Could you check a few things on this model? Use its own coordinates, in mm. A direction names the side the tool comes from. Coordinates: 2 decimals unless noted, no trailing zeros. Order: outer loops, then holes, each group sorted by start corner. A loop starts at its lowest first (then second) coordinate and runs counter-clockwise, first axis right, second up. Notation, with made-up numbers: M -8.5,46 L 34.5,46 A16 ccw 34.5,72 Z; hole C 85,56 d2. An arc over 180 degrees is marked long. Put each result on its own line as item: value. Start each with the question number.
```python
from build123d import *

# Parameters (mm, degrees)
AUFSATZ_LINEAR_AUSTRAGEN1_DEPTH      = 5
AUFSATZ_LINEAR_AUSTRAGEN2_DEPTH      = 1.25
AUFSATZ_LINEAR_AUSTRAGEN2_DEPTH_BACK = 1.25
SKIZZE2_W                            = 5
SKIZZE2_H                            = 5
SKIZZE3_R                            = 1.25
SCHNITT_LINEAR_AUSTRAGEN1_DEPTH      = 3.25
M3_GEWINDEBOHRUNG1_D                 = 2.5
M3_GEWINDEBOHRUNG1_DEPTH             = 8.5
M3_GEWINDEBOHRUNG1_TIP               = 0.751075774
VERRUNDUNG1_R                        = 2.5


with BuildPart() as part:
    # Skizze1 → Aufsatz-Linear austragen1 (new body)
    with BuildSketch(Plane.XY):
        with BuildLine():
            Line((-2.5, -3.535533906), (-2.5, -17.5))
            Line((-2.5, -17.5), (2.5, -17.5))
            Line((2.5, -17.5), (2.5, -3.535533906))
            ThreePointArc((2.5, -3.535533906), (2.622686042, -2.650995943), (2.981481481, -1.833239803))
            ThreePointArc((2.981481481, -1.833239803), (0, 3.5), (-2.981481481, -1.833239803))
            ThreePointArc((-2.981481481, -1.833239803), (-2.622686042, -2.650995943), (-2.5, -3.535533906))
        make_face()
    extrude(amount=AUFSATZ_LINEAR_AUSTRAGEN1_DEPTH)

    # Skizze2 → Aufsatz-Linear austragen2 (add, two sides: drawn at the far end of the back side and taken through both)
    with BuildSketch(Plane(origin=(0, 0, 0), x_dir=(0, 0, -1), z_dir=(1, 0, 0)).offset(-AUFSATZ_LINEAR_AUSTRAGEN2_DEPTH_BACK)):
        with Locations((-7.5, -15)):
            Rectangle(SKIZZE2_W, SKIZZE2_H)
    extrude(amount=AUFSATZ_LINEAR_AUSTRAGEN2_DEPTH + AUFSATZ_LINEAR_AUSTRAGEN2_DEPTH_BACK)

    # Skizze3 → Schnitt-Linear austragen1 (cut)
    with BuildSketch(Plane(origin=(1.25, 0, 0), x_dir=(0, 0, -1), z_dir=(1, 0, 0))):
        with Locations((-7.5, -15)):
            Circle(SKIZZE3_R)
    extrude(amount=-SCHNITT_LINEAR_AUSTRAGEN1_DEPTH, mode=Mode.SUBTRACT)

    # Skizze4 → Schnitt-Rotation1 (revolve, cut)
    with BuildSketch(Plane(origin=(0, 0, 0), x_dir=(1, 0, 0), z_dir=(0, 1, 0))):
        with BuildLine():
            Line((3, -5), (-3, -5))
            ThreePointArc((-3, -5), (0, -2), (3, -5))
        make_face()
    revolve(axis=Axis((7.725672482, 0, 5), (-1, 0, 0)), mode=Mode.SUBTRACT)

    # M3 Gewindebohrung1
    with Locations(Plane(origin=(0, -17.5, 2.5), x_dir=(0, 0, -1), z_dir=(0, -1, 0))):
        with Locations((0, 0)):
            Hole(M3_GEWINDEBOHRUNG1_D / 2, depth=M3_GEWINDEBOHRUNG1_DEPTH)
            with Locations((0, 0, -(M3_GEWINDEBOHRUNG1_DEPTH + M3_GEWINDEBOHRUNG1_TIP / 2))):  # 118° drill point
                Cone(0, M3_GEWINDEBOHRUNG1_D / 2, M3_GEWINDEBOHRUNG1_TIP, mode=Mode.SUBTRACT)

    # Verrundung1
    verrundung1_edges = [part.edges().sort_by_distance(p)[0] for p in [
        (0, -12.5, 5),
        (0, -12.5, 10),
        (0, -17.5, 10),
    ]]
    fillet(verrundung1_edges, radius=VERRUNDUNG1_R - 0.0001)  # a hair under: the kernel refuses the full size


solid = part.part
```
Item 1: If we section it at B-B on y = 0: Write out the boundary of the cut face in (x, z).
Item 2: For pin 1 Ø4 at (y, z) = (-8.5, 2.5) entering from -X; pin 2 Ø5 at (y, z) = (-7.5, 7) entering from +X; pin 3 Ø3 at (x, y) = (1, -4) entering from -Z; pin 4 Ø3 at (y, z) = (-15, 7.5) entering from -X, each with a flat end and sliding along its axis, tell me the tip position at first contact or that it passes through.
Item 3: I need wall thicknesses on probe 1 along Y at (x, z) = (-0.1, 7.5); probe 2 along X at (y, z) = (-11.5, 2.5); probe 3 along Z at (x, y) = (0, -14.5). Which ranges of each line are inside material? Lowest first, please.
Item 4: If we section it at C-C on y = -9.5: Write out the boundary of the cut face in (x, z).
Item 5: If we section it at A-A on z = 4.5: Write out the boundary of the cut face in (x, y), then the cut area to 3 significant figures.
Item 6: For faces 1 (the flat face through (0, -7, 5)), 2 (the flat face through (-1.25, -13.7, 6.98)), 3 (the flat face through (-2.5, -10, 2)), 4 (the cylindrical face through (0.38, -13.19, 3.69)), which set-ups out of +Z, -Z, +X, -X, +Y, -Y let a thin tool reach every point of the face, with its end or its side?
Item 7: If we mould it in two halves opening along Y, with no side actions, what happens to faces 5 (the flat face through (2.5, -11, 2)), 6 (the cylindrical face through (0.02, -13.76, 7.66)), 7 (the flat face through (1, -17.5, 4))? For each: released by +Y, released by -Y, zero draft, split by the parting line, or undercut.
Item 8: If we section it at D-D on y = -3.25: Write out the boundary of the cut face in (x, z).
Geometry check:
1. outline: M -3.5,0 L 3.5,0 L 3.5,5 L 3,5 A3 cw -3,5 L -3.5,5 Z
2. pin 1: stops at x = -2.5
2. pin 2: stops at x = 2.5
2. pin 3: stops at z = 0
2. pin 4: stops at x = -1.25
3. probe 1: y = -17.5 to -16.25, -13.75 to -12.5
3. probe 2: x = -2.5 to -1.25, 1.25 to 2.5
3. probe 3: z = 0 to 1.25, 3.75 to 6.35, 8.65 to 9.95
4. outline: M -2.5,0 L 2.5,0 L 2.5,5 L -2.5,5 Z; hole C 0,2.5 d2.5
5. outline: M -2.98,-1.83 A3.25 cw -2.5,-3.54 L -2.5,-17.5 L 2.5,-17.5 L 2.5,-3.54 A3.25 cw 2.98,-1.83 A3.5 ccw long Z; hole C 0,0 d5.92
5. area: 82.8 mm²
6. face 1: +Z, +Y
6. face 2: +Z, -X, +Y, -Y
6. face 3: +Z, -Z, -X, -Y
6. face 4: -Y
7. face 5: zero draft
7. face 6: undercut
7. face 7: released by -Y
8. outline: M -2.51,0 L 2.51,0 L 2.51,5 L -2.51,5 Z
